Model file for the job. Use its own axes, mm. A direction names the side the tool comes from. Round coordinates to 2 decimals unless told otherwise and drop trailing zeros. Order: outer loops, then holes, each group sorted by start corner. A loop starts at its lowest first (then second) coordinate and runs counter-clockwise, first axis right, second up. Notation, with made-up numbers: (25.5, -30) -> (48.5, -30) arc R24 cw to (48.5, -20) -> close; hole circle Ø11 at (4.5, 54). An arc over 180 degrees is marked (long way). Use CSV: the item, a comma, the result in double quotes.
```python
from build123d import *

# Parameters (mm, degrees)
BOSS_EXTRUDE1_DEPTH     = 25
SKETCH2_R               = 1.5
CUT_EXTRUDE1_DEPTH      = 1
CUT_EXTRUDE1_DEPTH_BACK = 12
CHAMFER1_SIZE           = 0.2
SKETCH4_R               = 1.5
BOSS_EXTRUDE2_DEPTH     = 6.5
CHAMFER2_SIZE           = 0.6


with BuildPart() as part:
    # Sketch1 → Boss-Extrude1 (new body)
    with BuildSketch(Plane.XY):
        Polygon((2.621170222, 0), (1.310585111, 2.27), (-1.310585111, 2.27), (-2.621170222, 0), (-1.310585111, -2.27), (1.310585111, -2.27), align=None)
    extrude(amount=BOSS_EXTRUDE1_DEPTH)

    # Sketch2 → Cut-Extrude1 (cut, two sides)
    with BuildSketch(Plane.XY.offset(25)) as cut_extrude1_sk:
        Circle(SKETCH2_R)
    extrude(amount=CUT_EXTRUDE1_DEPTH, mode=Mode.SUBTRACT)
    extrude(cut_extrude1_sk.sketch, amount=-CUT_EXTRUDE1_DEPTH_BACK, mode=Mode.SUBTRACT)

    # Sketch3 → Cut-Revolve1 (revolve, cut)
    with BuildSketch(Plane(origin=(0, 0, 0), x_dir=(1, 0, 0), z_dir=(0, 1, 0))):
        Polygon((-2.621170222, -25), (-2.271170222, -25), (-2.621170222, -24.8), align=None)
    revolve(axis=Axis((0, 0, 13), (0, 0, 1)), mode=Mode.SUBTRACT)

    # Chamfer1
    chamfer1_edges = [part.edges().sort_by_distance(p)[0] for p in [
        (-1.5, 0, 25),
    ]]
    chamfer(chamfer1_edges, length=CHAMFER1_SIZE)

    # Sketch4 → Boss-Extrude2 (add)
    with BuildSketch(Plane(origin=(0, 0, 0), x_dir=(-1, 0, 0), z_dir=(0, 0, -1))):
        Circle(SKETCH4_R)
    extrude(amount=BOSS_EXTRUDE2_DEPTH)

    # Chamfer2
    chamfer2_edges = [part.edges().sort_by_distance(p)[0] for p in [
        (1.5, 0, -6.5),
    ]]
    chamfer(chamfer2_edges, length=CHAMFER2_SIZE)


solid = part.part
```
Q1. Pin check, flat tip, straight feed: pin 1 (0.9 mm diameter, centred on x = -0.5, y = 0, fed in from +Z). Stop position of the tip, or through.
From the geometry:
pin 1,"stops at z = 13"
Q2. Mould opens along X. For faces 1 (the cylindrical face through (-1.5, 0.07, 18.98)), 2 (the flat face through (-1.975, -1.119, 12.325)), 3 (the flat face through (0, 0, 13)), 4 (the flat face through (1.957, -1.151, 12.325)) say: +X half, -X half, draft (parallel to the pull), parting line (faces both ways), or undercut.
From the geometry:
face 1,"undercut"
face 2,"-X half"
face 3,"undercut"
face 4,"+X half"
Q3. Cut at B-B (z = 3). Give the cut face in (x, y).
From the geometry:
outline,"(-2.62, 0) -> (-1.31, -2.27) -> (1.31, -2.27) -> (2.62, 0) -> (1.31, 2.27) -> (-1.31, 2.27) -> close"
Q4. Probe line 1 along Y through (x, z) = (0, 16.25); line 2 along Z through (x, y) = (0.3, -0.4); line 3 along Z through (x, y) = (-0.75, -1.8). List the from-to ranges inside material, lowest first.
From the geometry:
line 1,"y = -2.27 to -1.5, 1.5 to 2.27"
line 2,"z = -6.5 to 13"
line 3,"z = 0 to 25"
Q5. Cut at A-A (z = 23). Give the cut face in (x, y).
From the geometry:
outline,"(-2.62, 0) -> (-1.31, -2.27) -> (1.31, -2.27) -> (2.62, 0) -> (1.31, 2.27) -> (-1.31, 2.27) -> close; hole circle Ø3 at (0, 0)"
Q6. Cut at C-C (z = -0.5). Give the cut face in (x, y), plus the area to 3 significant figures.
From the geometry:
outline,"circle Ø3 at (0, 0)"
area,"7.07 mm²"
Q7. Which spindle directions (+Z, -Z, +X, -X, +Y, -Y) get a long thin tool onto all of the face, cutting with end or side? Do faces 5 (the flat face through (0, 2, 0)), 6 (the flat face through (0, -2.27, 12)). Say none if no direction does.
From the geometry:
face 5,"-Z"
face 6,"+Z, -Z, +X, -X, -Y"
